```python
from build123d import *

# Parameters (mm, degrees)
F0_W     = 86
F0_H     = 55
F1_DEPTH = 5
F2_W     = 80.25
F2_H     = 49.15
F3_DEPTH = 2
F4_R     = 2


with BuildPart() as f1:
    # F0 (on Top) → F1 (new body)
    with BuildSketch(Plane.XY):
        Rectangle(F0_W, F0_H)
    extrude(amount=F1_DEPTH)

    # F2 (on face) → F3 (cut)
    with BuildSketch(Plane.XY.offset(5)):
        with Locations((-0.125, -0.075)):
            Rectangle(F2_W, F2_H)
    extrude(amount=-F3_DEPTH, mode=Mode.SUBTRACT)

    # F4
    f4_edges = [f1.edges().sort_by_distance(p)[0] for p in [
        (-40.25, 24.5, 4),
        (-40.25, -24.65, 4),
        (40, 24.5, 4),
        (40, -24.65, 4),
    ]]
    fillet(f4_edges, radius=F4_R)


solid = f1.part
```
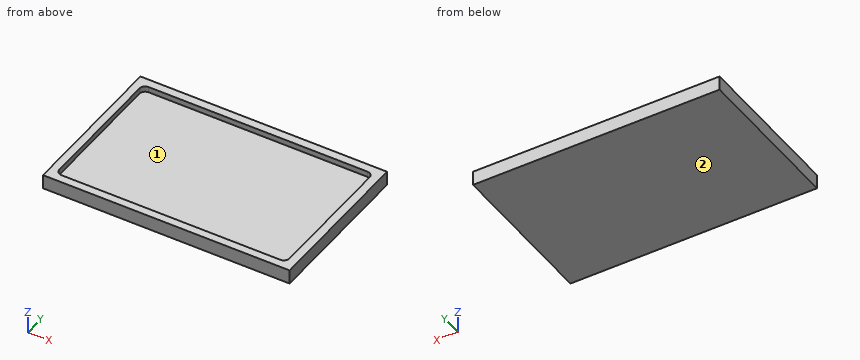
Build history of the part. All positions in model axes, mm. Face numbers are marked on the shaded views. Give positions to 0.01 mm unless a question says otherwise; leave off trailing zeros. Loops run counter-clockwise (first coordinate to the right, second up) from the corner with the lowest first, then second, coordinate; pieces in that order, holes last.
Item 1: Drill centre lines: line 1 (Y direction, x = -23, z = 3.6); line 2 (X direction, y = 14, z = 3.7); line 3 (Z direction, x = -7.5, y = -10). Where is each one in solid material? Low to high.
Answers follow:
line 1: y = -27.5 to -24.65, 24.5 to 27.5
line 2: x = -43 to -40.25, 40 to 43
line 3: z = 0 to 3
Item 2: Slice it at B-B, the plane x = 30. List the corners of the cut face in (y, z).
Answers follow:
outline: (-27.5, 0) - (27.5, 0) - (27.5, 5) - (24.5, 5) - (24.5, 3) - (-24.65, 3) - (-24.65, 5) - (-27.5, 5) - close
Item 3: Slice it at A-A, the plane z = 3.8. List the corners of the cut face in (x, y).
Answers follow:
outline: (-43, -27.5) - (43, -27.5) - (43, 27.5) - (-43, 27.5) - close; hole (-40.25, -22.65) arc R2 ccw to (-38.25, -24.65) - (38, -24.65) arc R2 ccw to (40, -22.65) - (40, 22.5) arc R2 ccw to (38, 24.5) - (-38.25, 24.5) arc R2 ccw to (-40.25, 22.5) - close
Item 4: Slice it at C-C, the plane y = -20. List the corners of the cut face in (x, z).
Answers follow:
outline: (-43, 0) - (43, 0) - (43, 5) - (40, 5) - (40, 3) - (-40.25, 3) - (-40.25, 5) - (-43, 5) - close
Item 5: Flat gauge pin, fed straight in: pin 1 (10 mm diameter, centred on x = 26.5, y = -14, fed in from +Z). Where does the tip first touch, or does it go through?
Answers follow:
pin 1: stops at z = 3
Item 6: Pull direction X, two halves, no side cores. Call the marked faces 1 and 2: released by +X, released by -X, zero draft, split by the parting line, or undercut.
Answers follow:
face 1: undercut
face 2: zero draft
